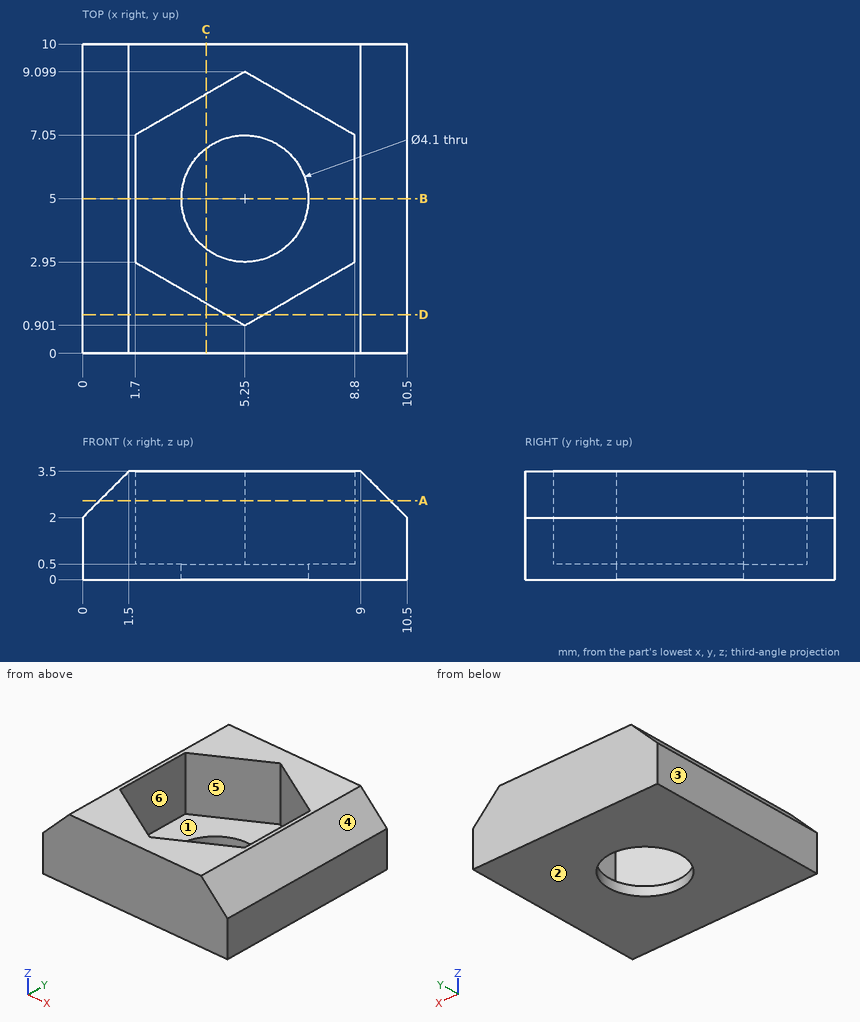
Verification items for this drawing (mm, ordinates from the low corner). A direction names the side the tool comes from. Round coordinates to 2 decimals unless told otherwise and drop trailing zeros. Order: outer loops, then holes, each group sorted by start corner. A loop starts at its lowest first (then second) coordinate and runs counter-clockwise, first axis right, second up.
1) Depth check by flat-ended pin: pin 1 (3.5 mm diameter, centred on x = 7, y = 5.5, fed in from +Z); pin 2 (2.5 mm diameter, centred on x = 5.25, y = 5, fed in from +Z). Enter the tip coordinate at first touch or a pass-through.
Geometry says:
pin 1: stops at z = 0.5
pin 2: passes through
2) Material ranges on line 1 (Y direction, x = 5.25, z = 0.2); line 2 (Y direction, x = 4.75, z = 1.9); line 3 (X direction, y = 6.5, z = 2.3), recorded low to high.
Geometry says:
line 1: y = 0 to 2.95, 7.05 to 10
line 2: y = 0 to 1.19, 8.81 to 10
line 3: x = 0.3 to 1.7, 8.8 to 10.2
3) Tool access check on the marked faces 1 and 2. Record the directions out of +Z, -Z, +X, -X, +Y, -Y that give a thin tool (end or side, any length) a straight path to the whole face; none if there is none.
Geometry says:
face 1: +Z
face 2: -Z, +X, -X, +Y, -Y
4) Cross-section at B-B, the plane y = 5. Record the cut outline in (x, z).
Geometry says:
outline: (0, 0) - (3.2, 0) - (3.2, 0.5) - (1.7, 0.5) - (1.7, 3.5) - (1.5, 3.5) - (0, 2) - close; (7.3, 0) - (10.5, 0) - (10.5, 2) - (9, 3.5) - (8.8, 3.5) - (8.8, 0.5) - (7.3, 0.5) - close
5) Cross-section at D-D, the plane y = 1.25. Record the cut outline in (x, z) (1 decimal).
Geometry says:
outline: (0, 0) - (10.5, 0) - (10.5, 2) - (9, 3.5) - (5.9, 3.5) - (5.9, 0.5) - (4.6, 0.5) - (4.6, 3.5) - (1.5, 3.5) - (0, 2) - close
6) Cross-section at C-C, the plane x = 4. Record the cut outline in (y, z) (1 decimal), plus the area to 3 significant figures.
Geometry says:
outline: (0, 0) - (3.4, 0) - (3.4, 0.5) - (1.6, 0.5) - (1.6, 3.5) - (0, 3.5) - close; (6.6, 0) - (10, 0) - (10, 3.5) - (8.4, 3.5) - (8.4, 0.5) - (6.6, 0.5) - close
area: 13.1 mm2
7) Cross-section at A-A, the plane z = 2.55. Record the cut outline in (x, y).
Geometry says:
outline: (0.55, 0) - (9.95, 0) - (9.95, 10) - (0.55, 10) - close; hole (1.7, 2.95) - (5.25, 0.9) - (8.8, 2.95) - (8.8, 7.05) - (5.25, 9.1) - (1.7, 7.05) - close
8) Draft check along X on the marked faces 3, 4, 5 and 6. Enter one of: +X half, -X half, draft (parallel to the pull), parting line (faces both ways), or undercut.
Geometry says:
face 3: -X half
face 4: +X half
face 5: undercut
face 6: undercut
